Here's how the part is built. I have some questions about the finished solid (model axes, mm). A direction names the side the tool comes from. Give positions to 0.01 mm unless a question says otherwise; leave off trailing zeros. Loops run counter-clockwise (first coordinate to the right, second up) from the corner with the lowest first, then second, coordinate; pieces in that order, holes last.
Q1. For faces 1 (the face through (-2, 0, 6)), 2 (the face through (0, 0.75, 2)), 3 (the face through (0, 0, 7)), which set-ups out of +Z, -Z, +X, -X, +Y, -Y let a thin tool reach every point of the face, with its end or its side?
Q2. Will these pins go through, and if not, where does the flat tip stop? P1, Ø1.5, axis at x = 1.5, z = 4.5, coming from the -Y side; P2, Ø2.5, axis at x = 0, z = 3.5, coming from the -Y side; P3, Ø1.4, axis at x = 1, z = 2, coming from the +Y side.
Q3. If we section it at B-B (z = 7.5): Please give me the cut outline in (x, y).
Q4. I need wall thicknesses on line 1 (Y direction, x = -0.1, z = 8); line 2 (Z direction, x = -1.1, y = 0.3); line 3 (Y direction, x = 0.5, z = 7.5). Which ranges of each line are inside material? Lowest first, please.
Q5. We'd pull the mould along Y, two halves only. Please class faces 4 (the face through (2.4, -0.09, 5.94)), 5 (the face through (0.016, -1.605, 11.661)), 6 (the face through (0.071, 1.603, 0.339)), 7 (the face through (0, -0.75, 10)): +Y half, -Y half, draft (parallel to the pull), parting line (faces both ways), or undercut.
Q6. If we section it at A-A (y = 0): Please give me the cut outline in (x, z), plus the area to 3 significant figures.
from build123d import *

# Parameters (mm, degrees)
F0_R         = 2.75
F1_DEPTH     = 2
F2_R         = 2.4
F3_DEPTH     = 8
F4_R         = 2.75
F5_DEPTH     = 2
F8_DEPTH     = 5
F10_DEPTH    = 5
F11_C1_SIZE2 = 1
F11_C1_SIZE  = 1.7320508076
F11_C2_SIZE2 = 1
F11_C2_SIZE  = 1.7320508076
F12_C1_SIZE2 = 1
F12_C1_SIZE  = 1.7320508076
F12_C2_SIZE2 = 1
F12_C2_SIZE  = 1.7320508076
F13_R        = 0.5
F15_DEPTH    = 25


# Not quite as in the source:
# - a fillet or chamfer that OpenCascade refuses, or shapes differently, is made with other operations: its cross-section is extruded or revolved along the edge and cut away or added


with BuildPart() as f1:
    # F0 (on Top) → F1 (new body)
    with BuildSketch(Plane.XY):
        Circle(F0_R)
    extrude(amount=F1_DEPTH)

    # F2 (on face) → F3 (join)
    with BuildSketch(Plane.XY.offset(2)):
        Circle(F2_R)
    extrude(amount=F3_DEPTH)

    # F4 (on face) → F5 (join)
    with BuildSketch(Plane.XY.offset(10)):
        Circle(F4_R)
    extrude(amount=F5_DEPTH)

    # F6: fillet of radius 0.5 on 2 edges, made by hand

    # F6_s1 → F6_t2 (revolve, cut)
    with BuildSketch(Plane.XZ):
        with BuildLine():
            ThreePointArc((2.4, 2), (2.6531128874, 1.8188343884), (2.75, 1.5230303993))
            Line((2.75, 1.5230303993), (2.75, 2))
            Line((2.75, 2), (2.4, 2))
        make_face()
    revolve(axis=Axis((0, 0, 2), (0, 0, 1)), mode=Mode.SUBTRACT)

    # F6_s3 → F6_t4 (revolve, cut)
    with BuildSketch(Plane.XZ):
        with BuildLine():
            ThreePointArc((2.75, 10.4769696007), (2.6531128874, 10.1811656116), (2.4, 10))
            Line((2.4, 10), (2.75, 10))
            Line((2.75, 10), (2.75, 10.4769696007))
        make_face()
    revolve(axis=Axis((0, 0, 10), (0, 0, 1)), mode=Mode.SUBTRACT)

    # F7 (on face) → F8 (cut)
    with BuildSketch(Plane(origin=(0, 0, 0), x_dir=(1, 0, 0), z_dir=(0, 0, -1))):
        with BuildLine():
            ThreePointArc((-2.6457513111, 0.75), (-2.75, 0), (-2.6457513111, -0.75))
            Line((-2.6457513111, -0.75), (2.6457513111, -0.75))
            ThreePointArc((2.6457513111, -0.75), (2.75, 0), (2.6457513111, 0.75))
            Line((2.6457513111, 0.75), (-2.6457513111, 0.75))
        make_face()
    extrude(amount=-F8_DEPTH, mode=Mode.SUBTRACT)

    # F9 (on face) → F10 (cut)
    with BuildSketch(Plane.XY.offset(12)):
        with BuildLine():
            ThreePointArc((-2.6457513111, 0.75), (-2.75, 0), (-2.6457513111, -0.75))
            Line((-2.6457513111, -0.75), (2.6457513111, -0.75))
            ThreePointArc((2.6457513111, -0.75), (2.75, 0), (2.6457513111, 0.75))
            Line((2.6457513111, 0.75), (-2.6457513111, 0.75))
        make_face()
    extrude(amount=-F10_DEPTH, mode=Mode.SUBTRACT)

    # F11: chamfer of 1 x 1.7320508076 on 2 edges, made by hand

    # F11_c1
    f11_c1_edges = [f1.edges().sort_by_distance(p)[0] for p in [
        (0, 2.75, 0),
    ]]
    f11_c1_side = f1.faces().sort_by_distance((0, 2.73, 0))[0]
    chamfer(f11_c1_edges, length=F11_C1_SIZE, length2=F11_C1_SIZE2, reference=f11_c1_side)

    # F11_c2
    f11_c2_edges = [f1.edges().sort_by_distance(p)[0] for p in [
        (0, -2.75, 0),
    ]]
    f11_c2_side = f1.faces().sort_by_distance((0, -2.73, 0))[0]
    chamfer(f11_c2_edges, length=F11_C2_SIZE, length2=F11_C2_SIZE2, reference=f11_c2_side)

    # F12: chamfer of 1 x 1.7320508076 on 2 edges, made by hand

    # F12_c1
    f12_c1_edges = [f1.edges().sort_by_distance(p)[0] for p in [
        (0, -2.75, 12),
    ]]
    f12_c1_side = f1.faces().sort_by_distance((0, -2.73, 12))[0]
    chamfer(f12_c1_edges, length=F12_C1_SIZE, length2=F12_C1_SIZE2, reference=f12_c1_side)

    # F12_c2
    f12_c2_edges = [f1.edges().sort_by_distance(p)[0] for p in [
        (0, 2.75, 12),
    ]]
    f12_c2_side = f1.faces().sort_by_distance((0, 2.73, 12))[0]
    chamfer(f12_c2_edges, length=F12_C2_SIZE, length2=F12_C2_SIZE2, reference=f12_c2_side)

    # F13
    f13_edges = [f1.edges().sort_by_distance(p)[0] for p in [
        (0, -2.75, 11),
        (0, 2.75, 11),
        (0, -2.75, 1),
        (0, 2.75, 1),
    ]]
    fillet(f13_edges, radius=F13_R)

    # F14 (on face) → F15 (cut)
    with BuildSketch(Plane.XY.offset(12)):
        with BuildLine():
            Line((-2, -1.8874586088), (-2, 1.8874586088))
            ThreePointArc((-2, 1.8874586088), (-2.75, 0), (-2, -1.8874586088))
        make_face()
    extrude(amount=-F15_DEPTH, mode=Mode.SUBTRACT)


solid = f1.part
Check sheet entries:
1. face 1: +Z, -Z, -X, +Y, -Y
1. face 2: -Z, +X, -X
1. face 3: +Z, +X, -X
2. P1: stops at y = -2.28
2. P2: stops at y = -2.4
2. P3: stops at y = 2.71
3. outline: (-2, -1.33) arc R2.4 ccw to (2.28, -0.75) - (-2, -0.75) - close; (-2, 0.75) - (2.28, 0.75) arc R2.4 ccw to (-2, 1.33) - close
4. line 1: y = -2.4 to -0.75, 0.75 to 2.4
4. line 2: z = 5 to 7
4. line 3: y = -2.35 to -0.75, 0.75 to 2.35
5. face 4: parting line
5. face 5: -Y half
5. face 6: +Y half
5. face 7: undercut
6. outline: (-2, 5) - (2.4, 5) - (2.4, 7) - (-2, 7) - close
6. area: 8.80 mm2
